Geometry check sheet. Reference: the model listing, model coordinates, mm. Face numbers are marked on the shaded views. Give positions to 0.01 mm unless a question says otherwise; leave off trailing zeros. Loops run counter-clockwise (first coordinate to the right, second up) from the corner with the lowest first, then second, coordinate; pieces in that order, holes last.
1. Release check for a two-part mould opening along X. For the marked faces 1, 2 and 3 record: +X half, -X half, draft (parallel to the pull), parting line (faces both ways), or undercut.
2. Go/stop test with flat-tipped pins: pin 1 Ø8 at (y, z) = (3.5, -15.5) entering from +X; pin 2 Ø1.7 at (y, z) = (23, -6) entering from +X; pin 3 Ø0.5 at (y, z) = (23.5, -3) entering from -X. Record where each tip stops, or that it passes through.
3. Cross-section at C-C, the plane y = 4.75. State how many separate pieces and enclosed holes the cut face has, plus the area to 3 significant figures.
4. Cross-section at B-B, the plane x = -5. Record the cut outline in (y, z), plus the area to 3 significant figures.
5. Cross-section at A-A, the plane z = -12. Record the cut outline in (x, y).
6. Material ranges on L1, parallel to X at y = 21.5, z = -20.5; L2, parallel to X at y = 19.5, z = 2.5; L3, parallel to Y at x = 7.5, z = -12.5, recorded low to high.
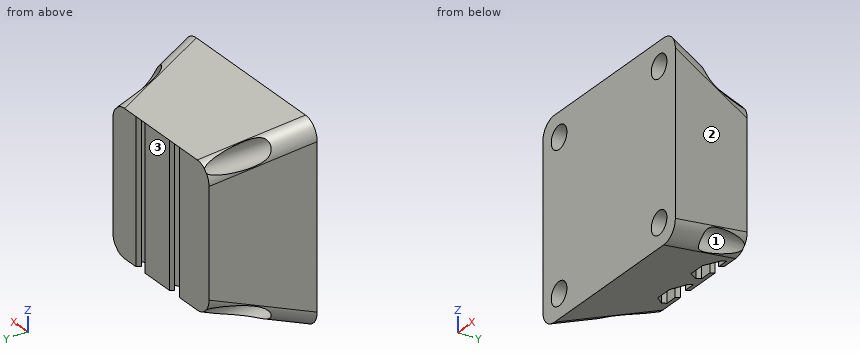
from build123d import *

# Parameters (mm, degrees)
SURFACE_FILL2_OUTLINE_W = 40
SURFACE_FILL2_OUTLINE_H = 40
SURFACE_FILL2_DEPTH     = 25.4
SURFACE_FILL2_DRAFT     = 16.595714
FILLET2_R               = 5.08
CUT_EXTRUDE3_DEPTH      = 47.53353416
CUT_EXTRUDE3_DEPTH_BACK = 47.53353416
SKETCH11_R              = 3.25
CUT_EXTRUDE4_START      = -41.921317507
CUT_EXTRUDE4_DEPTH      = 41.921317507


# Read off the part's stored shape, not the designer's step: Surface-Fill2, Cut-Extrude4
with BuildPart() as part:
    # Surface-Fill2 outline → Surface-Fill2 (with draft: the straight prism first)
    with BuildSketch(Plane(origin=(0, 25.4, 0), x_dir=(1, 0, 0), z_dir=(0, 1, 0))):
        Rectangle(SURFACE_FILL2_OUTLINE_W, SURFACE_FILL2_OUTLINE_H)
    extrude(amount=-SURFACE_FILL2_DEPTH)
    # Surface-Fill2: the draft: its side faces are tilted about the plane it starts from
    surface_fill2_sides = [part.faces().sort_by_distance(p)[0] for p in [
        (-20, 12.7, 0),
        (0, 12.7, 20),
        (20, 12.7, 0),
        (0, 12.7, -20),
    ]]
    draft(surface_fill2_sides, Plane(origin=(0, 25.4, 0), x_dir=(1, 0, 0), z_dir=(0, 1, 0)), SURFACE_FILL2_DRAFT)

    # Fillet2
    fillet2_edges = [part.edges().sort_by_distance(p)[0] for p in [
        (23.785000007, 12.7, -23.785000007),
        (23.785000007, 12.7, 23.785000007),
        (-23.785000007, 12.7, -23.785000007),
        (-23.785000007, 12.7, 23.785000007),
    ]]
    fillet(fillet2_edges, radius=FILLET2_R)

    # Sketch11 → Cut-Extrude3 (cut, two sides: drawn at the far end of the back side and taken through both)
    with BuildSketch(Plane(origin=(0, 0, 0), x_dir=(1, 0, 0), z_dir=(0, 1, 0)).offset(-CUT_EXTRUDE3_DEPTH_BACK)):
        with Locations(Location((-20.82, 20.82, 0), (0, 0, 326.308545858))):
            Circle(SKETCH11_R)
        with Locations(Location((20.82, 20.82, 0), (0, 0, 213.691454142))):
            Circle(SKETCH11_R)
        with Locations(Location((-20.82, -20.82, 0), (0, 0, 56.308545858))):
            Circle(SKETCH11_R)
        with Locations(Location((20.82, -20.82, 0), (0, 0, 123.691454142))):
            Circle(SKETCH11_R)
    extrude(amount=CUT_EXTRUDE3_DEPTH + CUT_EXTRUDE3_DEPTH_BACK, mode=Mode.SUBTRACT)

    # Cut-Extrude4 outline → Cut-Extrude4 (cut)
    with BuildSketch(Plane.XY.offset(20).offset(CUT_EXTRUDE4_START)):
        Polygon((13.737759609, 22.31), (13.737759609, 23.9), (10.367759609, 23.9), (10.367759609, 25.4), (6.679239208, 25.4), (6.679239208, 23.9), (3.309239208, 23.9), (3.309239208, 22.31), (6.138499409, 18.953307175), (10.908499409, 18.953307175), align=None)
        Polygon((-3.523215232, 23.9), (-3.523215232, 25.4), (-7.761612771, 25.4), (-7.761612771, 23.9), (-11.131612771, 23.9), (-11.131612771, 22.31), (-8.027414001, 19.205801231), (-3.257414001, 19.205801231), (-0.153215232, 22.31), (-0.153215232, 23.9), align=None)
    extrude(amount=CUT_EXTRUDE4_DEPTH, mode=Mode.SUBTRACT)


solid = part.part
Result:
1. face 1: undercut
1. face 2: +X half
1. face 3: draft
2. pin 1: stops at x = 27.57
2. pin 2: stops at x = 20.97
2. pin 3: stops at x = -20.64
3. separate pieces: 1
3. enclosed holes: 4
3. area: 2,580 mm2
4. outline: (0, -27.57) - (19.21, -21.85) - (19.21, 20) - (25.4, 20) - (0, 27.57) - close
4. area: 955 mm2
5. outline: (-27.57, 0) - (27.57, 0) - (20, 25.4) - (10.37, 25.4) - (10.37, 23.9) - (13.74, 23.9) - (13.74, 22.31) - (10.91, 18.95) - (6.14, 18.95) - (3.31, 22.31) - (3.31, 23.9) - (6.68, 23.9) - (6.68, 25.4) - (-3.52, 25.4) - (-3.52, 23.9) - (-0.15, 23.9) - (-0.15, 22.31) - (-3.26, 19.21) - (-8.03, 19.21) - (-11.13, 22.31) - (-11.13, 23.9) - (-7.76, 23.9) - (-7.76, 25.4) - (-20, 25.4) - close
6. L1: x = -17.59 to -10.32, -0.96 to 3.99, 13.06 to 17.59
6. L2: x = -21.76 to -8.32, -2.96 to 5.68, 11.37 to 21.76
6. L3: y = 0 to 18.95
